from build123d import *

# Parameters (mm, degrees)
BOSS_EXTRUDE1_DEPTH = 2
BOSS_EXTRUDE2_DEPTH = 30
SKETCH3_W           = 12
SKETCH3_H           = 40
BOSS_EXTRUDE3_DEPTH = 10
CUT_EXTRUDE1_DEPTH  = 35
SKETCH6_W           = 44
SKETCH6_H           = 23.882016553
CUT_EXTRUDE2_DEPTH  = 1
FILLET1_R           = 280
FILLET2_R           = 9
FILLET3_R           = 4
FILLET4_R           = 50


with BuildPart() as part:
    # Sketch1 → Boss-Extrude1 (new body)
    with BuildSketch(Plane(origin=(0, 0, 0), x_dir=(1, 0, 0), z_dir=(0, 1, 0))):
        Polygon((-27.5, 1.096246938), (-6, -38.903753062), (6, -38.903753062), (27.5, 1.096246938), (27.5, 41.096246938), (-27.5, 41.096246938), align=None)
    extrude(amount=BOSS_EXTRUDE1_DEPTH)

    # Sketch2 → Boss-Extrude2 (add)
    with BuildSketch(Plane(origin=(0, 2, 0), x_dir=(1, 0, 0), z_dir=(0, 1, 0))):
        Polygon((-22.5, 9.101662984), (-22.5, 34.101662984), (-12.65192247, 35.838144761), (-12.999218825, 37.807760267), (-24.816911861, 35.723982135), (-24.816911861, 7.479343833), (-12.999218825, 5.395565701), (-12.65192247, 7.365181207), align=None)
        Polygon((12.65192247, 7.365181207), (12.999218825, 5.395565701), (24.816911861, 7.479343833), (24.816911861, 35.723982135), (12.999218825, 37.807760267), (12.65192247, 35.838144761), (22.5, 34.101662984), (22.5, 9.101662984), align=None)
    extrude(amount=BOSS_EXTRUDE2_DEPTH)

    # Sketch3 → Boss-Extrude3 (add)
    with BuildSketch(Plane(origin=(0, 2, 0), x_dir=(1, 0, 0), z_dir=(0, 1, 0))):
        with Locations((-0.005517933, -18.7)):
            Rectangle(SKETCH3_W, SKETCH3_H)
    extrude(amount=BOSS_EXTRUDE3_DEPTH)

    # Sketch4 → Cut-Extrude1 (cut)
    with BuildSketch(Plane.XY.offset(38.7)):
        Polygon((0, 3.110912703), (3.889087297, 7), (0, 10.889087297), (-3.889087297, 7), align=None)
    extrude(amount=-CUT_EXTRUDE1_DEPTH, mode=Mode.SUBTRACT)

    # Sketch6 → Cut-Extrude2 (cut)
    with BuildSketch(Plane(origin=(0, 2, 0), x_dir=(1, 0, 0), z_dir=(0, 1, 0))):
        with Locations((0, 21.585626422)):
            Rectangle(SKETCH6_W, SKETCH6_H)
    extrude(amount=-CUT_EXTRUDE2_DEPTH, mode=Mode.SUBTRACT)

    # Fillet1
    # the kernel refuses this fillet: 280 mm, written as the material it adds along each edge
    with BuildSketch(Plane(origin=(22, 1, -92.634586786), x_dir=(0, 1, 0), z_dir=(0, 0, 1))) as fillet1_piece_1_section:
        with BuildLine():
            CenterArc((280, 23.643180835), FILLET1_R, 180, 4.843819526)
            Line((0, 23.643180835), (0, 0))
            Line((0, 0), (1, 0))
        make_face()
    fillet1_piece_1 = extrude(amount=142.097920729, mode=Mode.PRIVATE)
    fillet1_piece_1 = split(fillet1_piece_1, bisect_by=Plane(origin=(13.044676358, 1.194161729, -5.403581091), z_dir=(-0.17364817766692942, 0, -0.9848077530122082)), keep=Keep.TOP, mode=Mode.PRIVATE)
    fillet1_piece_1 = split(fillet1_piece_1, bisect_by=Plane(origin=(13.050161185, 1.194161729, -37.798777754), z_dir=(-0.1736481776669295, 0, 0.9848077530122082)), keep=Keep.TOP, mode=Mode.PRIVATE)
    add(fillet1_piece_1)
    with BuildSketch(Plane(origin=(-22, 1, -9.644618145), x_dir=(0, 1, 0), z_dir=(0, 0, -1))) as fillet1_piece_2:
        with BuildLine():
            CenterArc((280, 23.643180835), FILLET1_R, 180, 4.843819526)
            Line((0, 23.643180835), (0, 0))
            Line((0, 0), (1, 0))
        make_face()
    extrude(amount=23.882016554)

    # Fillet2
    fillet2_edges = [part.edges().sort_by_distance(p)[0] for p in [
        (-27.5, 1, -41.096246938),
        (27.5, 1, -41.096246938),
    ]]
    fillet(fillet2_edges, radius=FILLET2_R)

    # Fillet3
    # the kernel refuses this fillet: 4 mm, written as the material it takes off along each edge
    with BuildSketch(Plane(origin=(5.994482067, 12, 48.7), x_dir=(0, -1, 0), z_dir=(0, 0, -1)), Plane(origin=(-6.005517933, 12, -11.3), x_dir=(0, -1, 0), z_dir=(0, 0, 1))) as fillet3_piece_1:
        with BuildLine():
            CenterArc((FILLET3_R, FILLET3_R), FILLET3_R, 180, 90)
            Line((0, FILLET3_R), (0, 0))
            Line((0, 0), (FILLET3_R, 0))
        make_face()
    extrude(amount=60, mode=Mode.SUBTRACT)
    with BuildSketch(Plane(origin=(15.994482067, 12, -1.3), x_dir=(0, -1, 0), z_dir=(-1, 0, 0)), Plane(origin=(-16.005517933, 12, 38.7), x_dir=(0, -1, 0), z_dir=(1, 0, 0))) as fillet3_piece_2:
        with BuildLine():
            CenterArc((FILLET3_R, FILLET3_R), FILLET3_R, 180, 90)
            Line((0, FILLET3_R), (0, 0))
            Line((0, 0), (FILLET3_R, 0))
        make_face()
    extrude(amount=32, mode=Mode.SUBTRACT)

    # Fillet4
    fillet4_edges = [part.edges().sort_by_distance(p)[0] for p in [
        (-27.5, 1, -1.096246938),
        (27.5, 1, -1.096246938),
    ]]
    fillet(fillet4_edges, radius=FILLET4_R)


solid = part.part
Design review of the part built by this model. Coordinates are the model's own, in mm. A direction names the side the tool comes from. Round coordinates to 2 decimals unless told otherwise and drop trailing zeros. Loops run counter-clockwise (first coordinate to the right, second up) from the corner with the lowest first, then second, coordinate; pieces in that order, holes last. Notation, with made-up numbers: (-38.5, 44) -> (-22.5, 44) arc R22 ccw to (-22.5, 80) -> close; hole circle Ø3 at (42, 29). An arc over 180 degrees is marked (long way). Use one line per item in the form item = value. Start each with the question number.
Q1. Wall thickness on line 1 along X through (y, z) = (26, -33.5); line 2 along Y through (x, z) = (-11, 24); line 3 along Z through (x, y) = (15.5, 13): over which ranges is each line inside the solid? List them lowest first. Write a range as [from, to].
Q2. We need section A-A on y = 26. Give the boundary of the cut face in (x, z).
Q3. For pin 1 Ø14 at (y, z) = (21.5, -19) entering from -X; pin 2 Ø7.5 at (y, z) = (20.5, -24.5) entering from +X; pin 3 Ø1.8 at (y, z) = (4, 27) entering from +X, all flat-tipped, find the tip position at first contact; note any pin that passes through.
Q4. We need section D-D on z = 31.5. Give the boundary of the cut face in (x, y).
Q5. Machinability: for faces 4 (the face through (-0.09, 11.3, 36.96)), 5 (the face through (-24.817, 17, -22)), 6 (the face through (-1.97, 5.08, 21.45)), 7 (the face through (10.86, 1.28, -21.75)), 8 (the face through (27.5, 1, -23)), which of the approach directions +Z, -Z, +X, -X, +Y, -Y give a long, thin tool a straight path to every point of the face, cutting with its end or side? Answer none if there is none.
Q6. We need section B-B on z = -26. Give the boundary of the cut face in (x, y), then the cut area to 3 significant figures.
Q7. Draft analysis for pull direction Z (two halves, no side actions). For faces 1 (the face through (-27.5, 1, -23)), 2 (the face through (12.83, 16.79, -36.84)), 3 (the face through (-17.64, 16.79, -34.96)), state which applies: +Z half, -Z half, draft (parallel to the pull), parting line (faces both ways), or undercut.
Q8. We need section C-C on x = 15. Give the boundary of the cut face in (y, z), then the cut area to 3 significant figures.
Calculated:
q1.line_1 = [-24.82, -22.5], [22.5, 24.82]
q1.line_2 = [0, 2]
q1.line_3 = [-37.37, -35.34], [-7.87, -5.84]
q2.outline = (-24.82, -35.72) -> (-13, -37.81) -> (-12.65, -35.84) -> (-22.5, -34.1) -> (-22.5, -9.1) -> (-12.65, -7.37) -> (-13, -5.4) -> (-24.82, -7.48) -> close; (12.65, -35.84) -> (13, -37.81) -> (24.82, -35.72) -> (24.82, -7.48) -> (13, -5.4) -> (12.65, -7.37) -> (22.5, -9.1) -> (22.5, -34.1) -> close
q3.pin_1 = -24.82
q3.pin_2 = 24.82
q3.pin_3 = 5.99
q4.outline = (-9.98, 0) -> (9.98, 0) -> (9.98, 2) -> (5.99, 2) -> (5.99, 8) arc R4 ccw to (1.99, 12) -> (-2.01, 12) arc R4 ccw to (-6.01, 8) -> (-6.01, 2) -> (-9.98, 2) -> close; hole (-3.89, 7) -> (0, 3.11) -> (3.89, 7) -> (0, 10.89) -> close
q5.face_4 = +Z, +X, -X, +Y
q5.face_5 = +Z, -Z, -X, +Y
q5.face_6 = +Z
q5.face_7 = +Y
q5.face_8 = +Z, -Z, +X, +Y, -Y
q6.outline = (-27.5, 0) -> (27.5, 0) -> (27.5, 2) -> (24.82, 2) -> (24.82, 32) -> (22.5, 32) -> (22.5, 2) -> (22, 2) arc R280 cw to (0, 1) arc R280 cw to (-22, 2) -> (-22.5, 2) -> (-22.5, 32) -> (-24.82, 32) -> (-24.82, 2) -> (-27.5, 2) -> close
q6.area = 221 mm²
q7.face_1 = draft
q7.face_2 = -Z half
q7.face_3 = undercut
q8.outline = (0, -41.1) -> (2, -41.1) -> (2, -37.45) -> (32, -37.45) -> (32, -35.42) -> (2, -35.42) -> (2, -33.53) -> (1.5, -33.53) -> (1.5, -9.64) -> (2, -9.64) -> (2, -7.78) -> (32, -7.78) -> (32, -5.75) -> (2, -5.75) -> (2, 22.16) -> (0, 22.16) -> close
q8.area = 236 mm²
